For this review, use the dimensioned drawing (mm, ordinates from the lowest corner) and the shaded views. Coordinates: 2 decimals unless noted, no trailing zeros. Loops run counter-clockwise (first coordinate to the right, second up) from the corner with the lowest first, then second, coordinate; pieces in that order, holes last. Notation, with made-up numbers: M 61.25,51 L 86.25,51 A33 cw 86.25,89 Z; hole C 69,60.5 d5. An arc over 180 degrees is marked long. One line per item, written item: value.
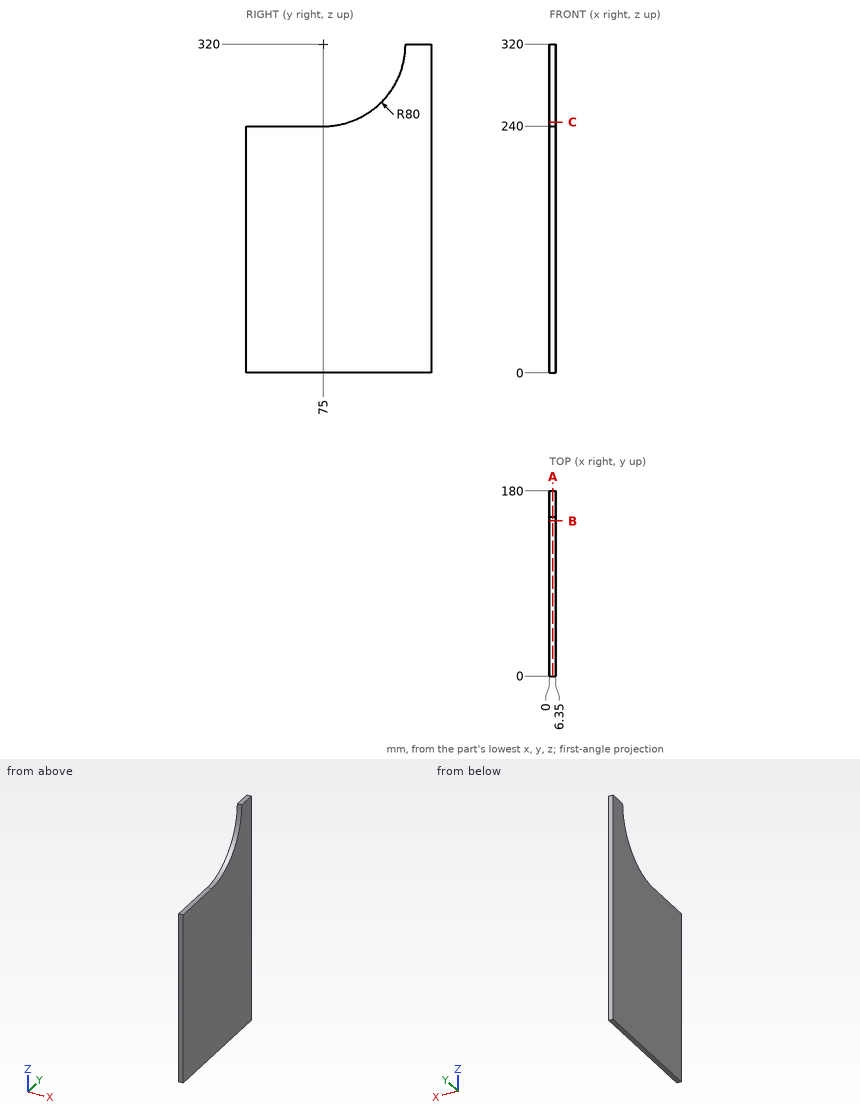
(1) We need section C-C on z = 244. State the section outline as (x, y) points.
Reply:
outline: M 0,99.98 L 6.35,99.98 L 6.35,180 L 0,180 Z
(2) We need section A-A on x = 3.5. State the section outline as (y, z) points.
Reply:
outline: M 0,0 L 180,0 L 180,320 L 155,320 A80 cw 75,240 L 0,240 Z
(3) We need section B-B on y = 151. State the section outline as (x, z) points, then the cut area to 3 significant figures.
Reply:
outline: M 0,0 L 6.35,0 L 6.35,295.02 L 0,295.02 Z
area: 1,870 mm2
(4) To check wall thickness, follow line 1 along Z through (x, y) = (0.75, 49.5); line 2 along Z through (x, y) = (2.75, 135.5); line 3 along Y through (x, z) = (5.25, 288). State the ranges of each line that lie inside material, in increasing order. Write a range as [from, to].
Reply:
line 1: z = [0, 240]
line 2: z = [0, 267.66]
line 3: y = [148.32, 180]
(5) Insertion check: pin 1 (12 mm diameter, centred on y = 99.5, z = 152, fed in from -X). The pin has a flat end and moves straight along its axis. Give the tip position at first contact, or say it passes through.
Reply:
pin 1: stops at x = 0
